Design review of the part built by this model. Coordinates are the model's own, in mm. A direction names the side the tool comes from. Give positions to 0.01 mm unless a question says otherwise; leave off trailing zeros. Answer as a JSON object with one key per item and string values.
from build123d import *

# Parameters (mm, degrees)
MASTER_SKETCH_R       = 52.451
MASTER_SKETCH_R_2     = 9.525
MASTER_SKETCH_R_3     = 45.974
MASTER_SKETCH_R_4     = 27.4955
MASTER_SKETCH_R_5     = 6.5
BOSS_EXTRUDE2_DEPTH   = 3.048
F_5_0MM_DOWEL_HOLE1_D = 5
CIRPATTERN4_COUNT     = 4
M6_CLEARANCE_HOLE4_D  = 6.6
M8_CLEARANCE_HOLE1_D  = 9
CIRPATTERN3_COUNT     = 18
CUT_EXTRUDE2_DEPTH    = 284.854467488
CUT_EXTRUDE4_DEPTH    = 284.854467488
FILLET1_R             = 3.175


with BuildPart() as part:
    # Master Sketch → Boss-Extrude2 (new, symmetric)
    # profile 1 of 5: a face of its own
    with BuildSketch(Plane(origin=(0, 0, 0), x_dir=(1, 0, 0), z_dir=(0, 1, 0))):
        with BuildLine():
            ThreePointArc((-8.636, 127), (-36.396097826, 84.787887478), (-86.152093601, 93.552952189))
            Line((-86.152093601, 93.552952189), (-6.534964144, 18.470363023))
            ThreePointArc((-6.534964144, 18.470363023), (-3.773598517, 34.145603423), (9.525, 25.4))
            ThreePointArc((9.525, 25.4), (8.799952547, 21.754940307), (6.735192091, 18.664807909))
            Line((6.735192091, 18.664807909), (34.255961574, 46.185577392))
            ThreePointArc((34.255961574, 46.185577392), (59.945142207, 60.02346539), (89.010077776, 57.44457682))
            Line((89.010077776, 57.44457682), (207.987004211, 9.951947906))
            ThreePointArc((207.987004211, 9.951947906), (204.851852042, 25.601533276), (220.43444462, 22.148779315))
            Line((220.43444462, 22.148779315), (189.133864847, 105.44289655))
            ThreePointArc((189.133864847, 105.44289655), (188.207777178, 115.4635324), (192.51641215, 124.557840832))
            Line((192.51641215, 124.557840832), (212.800120602, 148.168522003))
            ThreePointArc((212.800120602, 148.168522003), (196.940842995, 150.353698677), (205.472725722, 163.899866417))
            Line((205.472725722, 163.899866417), (169.599038165, 163.514054819))
            ThreePointArc((169.599038165, 163.514054819), (163.800537316, 164.352688386), (158.531122559, 166.913779261))
            ThreePointArc((158.531122559, 166.913779261), (141.706259737, 175.147152322), (123.19, 177.9778))
            Line((123.19, 177.9778), (-54.61, 172.974))
            ThreePointArc((-54.61, 172.974), (-22.101472842, 159.508527158), (-8.636, 127))
        make_face()
        with Locations(Location((123.19, 116.0018, 0), (0, 0, 90))):
            Circle(MASTER_SKETCH_R, mode=Mode.SUBTRACT)
    # profile 2 of 5: a face of its own
    with BuildSketch(Plane(origin=(0, 0, 0), x_dir=(1, 0, 0), z_dir=(0, 1, 0))):
        with Locations((0, 25.4)):
            Circle(MASTER_SKETCH_R_2)
    # profile 3 of 5: a face of its own
    with BuildSketch(Plane(origin=(0, 0, 0), x_dir=(1, 0, 0), z_dir=(0, 1, 0))):
        with Locations((211.518208908, 18.79820239)):
            Circle(MASTER_SKETCH_R_2)
    # profile 4 of 5: a face of its own
    with BuildSketch(Plane(origin=(0, 0, 0), x_dir=(1, 0, 0), z_dir=(0, 1, 0))):
        with Locations((205.575158542, 154.375417219)):
            Circle(MASTER_SKETCH_R_2)
    # profile 5 of 5: a face of its own
    with BuildSketch(Plane(origin=(0, 0, 0), x_dir=(1, 0, 0), z_dir=(0, 1, 0))):
        with Locations((-54.61, 127)):
            Circle(MASTER_SKETCH_R_3)
        with Locations(Location((-54.61, 127, 0), (0, 0, 90))):
            Circle(MASTER_SKETCH_R_4, mode=Mode.SUBTRACT)
        with Locations(Location((-41.27121441, 90.351987789, 0), (0, 0, 90))):
            Circle(MASTER_SKETCH_R_5, mode=Mode.SUBTRACT)
        with Locations(Location((-67.94878559, 90.351987789, 0), (0, 0, 90))):
            Circle(MASTER_SKETCH_R_5, mode=Mode.SUBTRACT)
    extrude(amount=BOSS_EXTRUDE2_DEPTH, both=True)

    # Ø5.0mm Dowel Hole1 (through all)
    with Locations(Plane(origin=(0, 3.048, 0), x_dir=(1, 0, 0), z_dir=(0, 1, 0))):
        with Locations((123.19, 173.1518)):
            f_5_0mm_dowel_hole1 = Hole(F_5_0MM_DOWEL_HOLE1_D / 2)

    # CirPattern4: Ø5.0mm Dowel Hole1 ×4 about axis
    cirpattern4_axis = Axis((123.19, 0, -116.0018), (0, 1, 0))
    for i in range(1, CIRPATTERN4_COUNT):
        add(f_5_0mm_dowel_hole1.rotate(cirpattern4_axis, i * 360 / CIRPATTERN4_COUNT), mode=Mode.SUBTRACT)

    # M6 Clearance Hole4 (through all)
    with Locations(Plane(origin=(0, 3.048, 0), x_dir=(1, 0, 0), z_dir=(0, 1, 0))):
        with Locations((205.575158542, 154.375417219), (211.518208908, 18.79820239), (0, 25.4)):
            Hole(M6_CLEARANCE_HOLE4_D / 2)

    # M8 Clearance Hole1 (through all)
    with Locations(Plane(origin=(0, 3.048, 0), x_dir=(1, 0, 0), z_dir=(0, 1, 0))):
        with Locations((-54.61, 166)):
            m8_clearance_hole1 = Hole(M8_CLEARANCE_HOLE1_D / 2)

    # CirPattern3: M8 Clearance Hole1 ×18 about axis, 10 skipped
    cirpattern3_axis = Axis((-54.61, 3.048, -127), (0, -1, 0))
    add([m8_clearance_hole1.rotate(cirpattern3_axis, i * 360 / CIRPATTERN3_COUNT) for i in range(1, CIRPATTERN3_COUNT) if i not in (1, 3, 5, 7, 8, 10, 11, 13, 15, 17)], mode=Mode.SUBTRACT)

    # Topology 3 → Cut-Extrude2 (cut, through all)
    with BuildSketch(Plane(origin=(0, 3.048, 0), x_dir=(1, 0, 0), z_dir=(0, 1, 0))):
        with BuildLine():
            Line((148.232551201, 44.060262413), (194.821264757, 25.463207079))
            ThreePointArc((194.821264757, 25.463207079), (203.319232726, 27.16564341), (205.194131764, 35.627233252))
            Line((205.194131764, 35.627233252), (188.900120968, 78.987300553))
            ThreePointArc((188.900120968, 78.987300553), (183.658143307, 83.064639882), (177.648151764, 80.239214699))
            ThreePointArc((177.648151764, 80.239214699), (164.735029841, 65.81551406), (148.153589294, 55.823132596))
            ThreePointArc((148.153589294, 55.823132596), (144.236830733, 49.915140022), (148.232551201, 44.060262413))
        make_face()
        with BuildLine():
            Line((188.044823271, 154.186883307), (181.870154841, 154.120476454))
            ThreePointArc((181.870154841, 154.120476454), (179.135815493, 152.500048502), (179.17593949, 149.321874737))
            ThreePointArc((179.17593949, 149.321874737), (182.248718341, 143.510354832), (184.720207534, 137.418764347))
            ThreePointArc((184.720207534, 137.418764347), (187.127250613, 135.343061567), (190.127076346, 136.393510988))
            Line((190.127076346, 136.393510988), (194.150985671, 141.077429629))
            ThreePointArc((194.150985671, 141.077429629), (195.32544691, 149.601274428), (188.044823271, 154.186883307))
        make_face()
        with BuildLine():
            Line((17.44176984, 42.84176984), (27.520769483, 52.920769483))
            ThreePointArc((27.520769483, 52.920769483), (42.409632623, 63.819008448), (59.896219631, 69.707058463))
            ThreePointArc((59.896219631, 69.707058463), (66.885503662, 75.024623751), (66.553177874, 83.800508404))
            ThreePointArc((66.553177874, 83.800508404), (62.745475764, 91.688999032), (60.030376503, 100.016970919))
            ThreePointArc((60.030376503, 100.016970919), (55.6852269, 105.854731176), (48.48636159, 106.920614917))
            Line((48.48636159, 106.920614917), (-7.457826773, 92.934567826))
            ThreePointArc((-7.457826773, 92.934567826), (-16.98904431, 89.126755018), (-25.157987823, 82.912906934))
            Line((-25.157987823, 82.912906934), (-33.299725858, 74.771168898))
            ThreePointArc((-33.299725858, 74.771168898), (-37.018106584, 65.604842248), (-33.032755262, 56.551396808))
            Line((-33.032755262, 56.551396808), (-17.945313453, 42.323250142))
            ThreePointArc((-17.945313453, 42.323250142), (-0.146601343, 35.405008389), (17.44176984, 42.84176984))
        make_face()
        with BuildLine():
            Line((60.61677272, 166.688039353), (-1.663792567, 164.935286301))
            ThreePointArc((-1.663792567, 164.935286301), (-9.632748017, 160.197249287), (-9.798074059, 150.927626155))
            ThreePointArc((-9.798074059, 150.927626155), (-6.09260405, 142.056636088), (-4.12477238, 132.646396384))
            ThreePointArc((-4.12477238, 132.646396384), (-0.093621954, 125.882803807), (7.651359628, 124.464488392))
            Line((7.651359628, 124.464488392), (55.659374127, 136.466492017))
            ThreePointArc((55.659374127, 136.466492017), (60.668494681, 138.996854714), (64.098067009, 143.438932802))
            ThreePointArc((64.098067009, 143.438932802), (66.306808777, 147.765857633), (68.831828447, 151.916170194))
            ThreePointArc((68.831828447, 151.916170194), (69.209050275, 161.796201373), (60.61677272, 166.688039353))
        make_face()
    extrude(amount=-CUT_EXTRUDE2_DEPTH, mode=Mode.SUBTRACT)

    # Sketch29 → Cut-Extrude4 (cut, through all)
    with BuildSketch(Plane(origin=(0, 3.048, 0), x_dir=(1, 0, 0), z_dir=(0, 1, 0))):
        with BuildLine():
            Line((-74.056787625, 92.575118721), (-76.882563864, 84.811362311))
            Line((-76.882563864, 84.811362311), (-66.583357956, 75.098740778))
            Line((-66.583357956, 75.098740778), (-61.840783555, 88.128856858))
            ThreePointArc((-61.840783555, 88.128856858), (-70.171916521, 84.243985754), (-74.056787625, 92.575118721))
        make_face()
    extrude(amount=-CUT_EXTRUDE4_DEPTH, mode=Mode.SUBTRACT)

    # Fillet1
    fillet1_edges = [part.edges().sort_by_distance(p)[0] for p in [
        (-66.583357956, 0, -75.098740778),
        (-76.882563864, 0, -84.811362311),
    ]]
    fillet(fillet1_edges, radius=FILLET1_R)


solid = part.part
(1) We need section A-A (y = 0). Count the separate pieces of the cut face and the enclosed holes in it, plus the area to 3 significant figures.
Checked values:
{"separate pieces": "1", "enclosed holes": "22", "area": "16,800 mm^2"}
(2) Insertion check: pin 1 (1 mm diameter, centred on x = 136.5, y = -1, fed in from +Z); pin 2 (5.5 mm diameter, centred on x = -16.2, z = -133.77, fed in from +Y). Each pin has a flat end and moves straight along its axis. Give the tip position at first contact, or say it passes through.
Checked values:
{"pin 1": "stops at z = -38.29", "pin 2": "passes through"}
(3) To check wall thickness, follow L1, parallel to Z at x = 51, y = 2.75; L2, parallel to Z at x = -14, y = -2.25; L3, parallel to Z at x = 67, y = -2.5. State the ranges of each line that lie inside material, in increasing order. Write a range as from..to.
Checked values:
{"L1": "z = -175.95..-166.42, -135.3..-107.2, -67.46..-57.31", "L2": "z = -174.12..-137.7, -129.85..-90.65, -39.28..-25.51", "L3": "z = -176.4..-164.47, -148.98..-118.31, -113.69..-82.91, -75.28..-60.97"}
(4) Draft analysis for pull direction Z (two halves, no side actions). For faces 3 (the cylindrical face through (141.957, -0.043, -175.068)), 4 (the flat face through (-36.209, 0.043, -46.454)), 5 (the cylindrical face through (-6.133, 0.043, -142.185)), state which applies: +Z half, -Z half, draft (parallel to the pull), parting line (faces both ways), or undercut.
Checked values:
{"face 3": "-Z half", "face 4": "+Z half", "face 5": "undercut"}
(5) Tool access review of faces 1 (the flat face through (197.161, 0.043, -57.004)), 2 (the flat face through (59, 3.048, -113)): name each direction out of +Z, -Z, +X, -X, +Y, -Y from which nothing blocks a thin tool from reaching the whole face with its end or side.
Checked values:
{"face 1": "+Y, -Y", "face 2": "+Z, -Z, +X, -X, +Y"}
